CAD build for the part. Positions are in the model's coordinates, mm. A direction names the side the tool comes from. Give positions to 0.01 mm unless a question says otherwise; leave off trailing zeros. Loops run counter-clockwise (first coordinate to the right, second up) from the corner with the lowest first, then second, coordinate; pieces in that order, holes last.
Item 1: Saw through at A-A on y = 10. Give the cut face in (x, z).
Item 2: Drop flat-ended pins along their axis: P1, Ø2, axis at y = 32, z = 3, coming from the +X side; P2, Ø3, axis at x = 0, z = 0, coming from the -Y side; P3, Ø1.5, axis at x = 1, z = 1, coming from the +Y side. Give the stop position or say it passes through.
Item 3: Which spindle directions (+Z, -Z, +X, -X, +Y, -Y) get a long thin tool onto all of the face, cutting with end or side? Do faces 1 (the flat face through (-4, 22, 3.5)), 2 (the flat face through (-4.348, 9.628, 2.469)), 3 (the flat face through (-4.312, 9.628, -2.531)), 4 (the flat face through (4.348, 9.628, -2.469)), 5 (the flat face through (4.312, 9.628, 2.531)). Say none if no direction does.
Item 4: Mould opens along Z. For faces 6 (the flat face through (0, 8, 5)), 7 (the flat face through (0, 21, -3.5)), 8 (the cylindrical face through (2.345, 6.93, -0.738)) say: released by +Z, released by -Z, zero draft, split by the parting line, or undercut.
Item 5: Probe probe 1 along X at (y, z) = (6.75, 0); probe 2 along Z at (x, y) = (0, 6.5); probe 3 along Y at (x, z) = (-3.75, 0.75). List the from-to ranges inside material, lowest first.
from build123d import *

# Parameters (mm, degrees)
BOSS_EXTRUDE1_DEPTH     = 30
CUT_EXTRUDE1_DEPTH      = 11
CUT_EXTRUDE1_DEPTH_BACK = 11


with BuildPart() as part:
    # Sketch1 → Boss-Extrude1 (new body)
    with BuildSketch(Plane(origin=(0, 0, 0), x_dir=(1, 0, 0), z_dir=(0, 1, 0))):
        with BuildLine():
            Line((-5.624045, -0.258867), (-3.036209, -4.741133))
            ThreePointArc((-3.036209, -4.741133), (-2.815, -4.875723), (-2.587837, -5))
            Line((-2.587837, -5), (2.587837, -5))
            ThreePointArc((2.587837, -5), (2.815, -4.875723), (3.036209, -4.741133))
            Line((3.036209, -4.741133), (5.624045, -0.258867))
            ThreePointArc((5.624045, -0.258867), (5.63, 0), (5.624045, 0.258867))
            Line((5.624045, 0.258867), (3.036209, 4.741133))
            ThreePointArc((3.036209, 4.741133), (2.815, 4.875723), (2.587837, 5))
            Line((2.587837, 5), (-2.587837, 5))
            ThreePointArc((-2.587837, 5), (-2.815, 4.875723), (-3.036209, 4.741133))
            Line((-3.036209, 4.741133), (-5.624045, 0.258867))
            ThreePointArc((-5.624045, 0.258867), (-5.63, 0), (-5.624045, -0.258867))
        make_face()
    extrude(amount=BOSS_EXTRUDE1_DEPTH)

    # Sketch2 → Revolve1 (revolve)
    with BuildSketch(Plane.XY):
        with BuildLine():
            Line((8.746197, 25.151904), (0, 9.373347))
            Line((0, 9.373347), (0, 40))
            ThreePointArc((0, 40), (8.616292, 35.075384), (8.746197, 25.151904))
        make_face()
    revolve(axis=Axis((0, 9.373347, 0), (0, 1, 0)))

    # Sketch3 → Cut-Extrude1 (cut, two sides)
    with BuildSketch(Plane(origin=(0, 0, 0), x_dir=(0, 0, -1), z_dir=(1, 0, 0))) as cut_extrude1_sk:
        Polygon((-11, 10), (-7.746665, 10), (-3.5, 20.004517), (-3.5, 40), (3.5, 40), (3.5, 20.004517), (7.746665, 10), (11, 10), (11, 50), (-11, 50), align=None)
    extrude(amount=CUT_EXTRUDE1_DEPTH, mode=Mode.SUBTRACT)
    extrude(cut_extrude1_sk.sketch, amount=-CUT_EXTRUDE1_DEPTH_BACK, mode=Mode.SUBTRACT)

    # Sketch4 → Cut-Revolve1 (revolve, cut)
    with BuildSketch(Plane.XY):
        Polygon((0, 14.919416), (2.4585, 13.5), (2.4585, 0.5415), (3, 0), (0, 0), align=None)
    revolve(axis=Axis((0, 0, 0), (0, 1, 0)), mode=Mode.SUBTRACT)

    # Sketch5 → Cut-Revolve2 (revolve, cut)
    with BuildSketch(Plane(origin=(0, 0, 0), x_dir=(0, 0, -1), z_dir=(1, 0, 0))):
        with BuildLine():
            Line((-4.5, 30), (-4.5, 38.6))
            Line((-4.5, 38.6), (-3.5, 38.6))
            Line((-3.5, 38.6), (-2.376818, 35.888398))
            ThreePointArc((-2.376818, 35.888398), (0, 36.35), (2.376818, 35.888398))
            Line((2.376818, 35.888398), (3.5, 38.6))
            Line((3.5, 38.6), (4.5, 38.6))
            Line((4.5, 38.6), (4.5, 30))
            Line((4.5, 30), (-4.5, 30))
        make_face()
    revolve(axis=Axis((0, 30, -4.5), (0, 0, 1)), mode=Mode.SUBTRACT)


solid = part.part
Results below:
1. outline: (-5.62, -0.26) - (-3.04, -4.74) arc R5.63 ccw to (-2.59, -5) - (2.59, -5) arc R5.63 ccw to (3.04, -4.74) - (5.62, -0.26) arc R5.63 ccw to (5.62, 0.26) - (3.04, 4.74) arc R5.63 ccw to (2.59, 5) - (-2.59, 5) arc R5.63 ccw to (-3.04, 4.74) - (-5.62, 0.26) arc R5.63 ccw to start; hole circle Ø4.92 at (0, 0)
2. P1: stops at x = 9.65
2. P2: stops at y = 14.05
2. P3: stops at y = 39.98
3. face 1: +Z, +X, -X, +Y
3. face 2: +Z, -X, -Y
3. face 3: -Z, -X, -Y
3. face 4: -Z, +X, -Y
3. face 5: +Z, +X, -Y
4. face 6: released by +Z
4. face 7: released by -Z
4. face 8: undercut
5. probe 1: x = -5.63 to -2.46, 2.46 to 5.63
5. probe 2: z = -5 to -2.46, 2.46 to 5
5. probe 3: y = 0 to 24.93, 35.07 to 39.24
